Could you check a few things on this model? Use its own coordinates, in mm. A direction names the side the tool comes from. Give positions to 0.01 mm unless a question says otherwise; leave off trailing zeros. Order: outer loops, then holes, each group sorted by start corner. A loop starts at its lowest first (then second) coordinate and runs counter-clockwise, first axis right, second up. Notation, with made-up numbers: (5.5, 78) - (53.5, 78) arc R28 ccw to (53.5, 104) - close; hole circle Ø6 at (-9.75, -21). An arc over 180 degrees is marked (long way). One line per question, with ' | ' between items. Start each with the question number.
1. Imagine slicing it at B-B (x = 8). Please give me the cut outline in (y, z), and give its area (3 significant figures).
2. Imagine slicing it at A-A (z = -12). Please give me the cut outline in (x, y) (3 decimals).
3. I need wall thicknesses on probe 1 along Z at (x, y) = (3, -39); probe 2 along Y at (x, z) = (8.75, 7). Which ranges of each line are inside material? Lowest first, please. Write a range as from..to.
4. Imagine slicing it at C-C (y = -10.5). Please give me the cut outline in (x, z) (1 decimal), and give its area (3 significant figures).
5. Which directions (+Z, -Z, +X, -X, +Y, -Y) give clear straight access to the entire face, cutting with the end or side of a thin tool? Please do faces 1 (the cylindrical face through (4.696, 86.99, -63.277)), 2 (the flat face through (5, 82.55, 1)).
6. If we mould it in two halves opening along Z, with no side actions, what happens to faces 3 (the cylindrical face through (4.7, -87.09, -63.18)), 4 (the flat face through (9.525, -7, -62)), 5 (the flat face through (5, 1, -58.738))? For each: released by +Z, released by -Z, zero draft, split by the parting line, or undercut.
```python
from build123d import *

# Parameters (mm, degrees)
F1_DEPTH = 9.525


# Not quite as in the source:
# - a length typed as a fraction of an inch, garbled in the dataset ("3 / 203.2 mm" for 3/8 in), is restored


with BuildPart() as f1:
    # F0 (on Right) → F1 (new body)
    with BuildSketch(Plane.YZ):
        with BuildLine():
            ThreePointArc((88.9, 58.7375), (87.0401280605, 63.2276280605), (82.55, 65.0875))
            Line((82.55, 65.0875), (-82.55, 65.0875))
            ThreePointArc((-82.55, 65.0875), (-87.0401280605, 63.2276280605), (-88.9, 58.7375))
            Line((-88.9, 58.7375), (-88.9, -58.7375))
            ThreePointArc((-88.9, -58.7375), (-87.0401280605, -63.2276280605), (-82.55, -65.0875))
            Line((-82.55, -65.0875), (82.55, -65.0875))
            ThreePointArc((82.55, -65.0875), (87.0401280605, -63.2276280605), (88.9, -58.7375))
            Line((88.9, -58.7375), (88.9, 58.7375))
        make_face()
        Polygon((82.55, 58.7375), (82.55, 53.975), (82.55, -53.975), (82.55, -58.7375), (74.6125, -58.7375), (-74.6125, -58.7375), (-82.55, -58.7375), (-82.55, -53.975), (-82.55, 53.975), (-82.55, 58.7375), (-74.6125, 58.7375), (74.6125, 58.7375), align=None, mode=Mode.SUBTRACT)
    extrude(amount=F1_DEPTH)


solid = f1.part
```
Results found:
1) outline: (-88.9, -58.74) arc R6.35 ccw to (-82.55, -65.09) - (82.55, -65.09) arc R6.35 ccw to (88.9, -58.74) - (88.9, 58.74) arc R6.35 ccw to (82.55, 65.09) - (-82.55, 65.09) arc R6.35 ccw to (-88.9, 58.74) - close; hole (-82.55, -58.74) - (82.55, -58.74) - (82.55, 58.74) - (-82.55, 58.74) - close | area: 3,720 mm2
2) outline: (0, -88.9) - (9.525, -88.9) - (9.525, -82.55) - (0, -82.55) - close; (0, 82.55) - (9.525, 82.55) - (9.525, 88.9) - (0, 88.9) - close
3) probe 1: z = -65.09..-58.74, 58.74..65.09 | probe 2: y = -88.9..-82.55, 82.55..88.9
4) outline: (0, -65.1) - (9.5, -65.1) - (9.5, -58.7) - (0, -58.7) - close; (0, 58.7) - (9.5, 58.7) - (9.5, 65.1) - (0, 65.1) - close | area: 121 mm2
5) face 1: -Z, +X, -X, +Y | face 2: +X, -X
6) face 3: released by -Z | face 4: zero draft | face 5: undercut
